```python
from build123d import *

# Parameters (mm, degrees)
SKETCH2_W     = 2.75
SKETCH2_H     = 10
CHAMFER1_SIZE = 3
CHAMFER2_SIZE = 1


with BuildPart() as part:
    # Sketch2 → Revolve1 (revolve)
    with BuildSketch(Plane(origin=(0, 0, 0), x_dir=(0, 0, -1), z_dir=(1, 0, 0))):
        Polygon((14.3, 12), (14.3, 0), (17.05, 0), (23.05, 0), (23.05, 12), align=None)
        with Locations((15.675, -5)):
            Rectangle(SKETCH2_W, SKETCH2_H)
    revolve(axis=Axis((0, -11.25, 0), (0, 1, 0)))

    # Chamfer1
    chamfer1_edges = [part.edges().sort_by_distance(p)[0] for p in [
        (0, 12, 23.05),
        (0, 0, 23.05),
    ]]
    chamfer(chamfer1_edges, length=CHAMFER1_SIZE)

    # Chamfer2
    chamfer2_edges = [part.edges().sort_by_distance(p)[0] for p in [
        (0, -10, 17.05),
    ]]
    chamfer(chamfer2_edges, length=CHAMFER2_SIZE)


solid = part.part
```
Build history of the part. All positions in model axes, mm. A direction names the side the tool comes from. Give positions to 0.01 mm unless a question says otherwise; leave off trailing zeros. Loops run counter-clockwise (first coordinate to the right, second up) from the corner with the lowest first, then second, coordinate; pieces in that order, holes last.
Item 1: Slice it at B-B, the plane x = 0. List the corners of the cut face in (y, z).
Answers follow:
outline: (-10, -16.05) - (-9, -17.05) - (0, -17.05) - (0, -20.05) - (3, -23.05) - (9, -23.05) - (12, -20.05) - (12, -14.3) - (-10, -14.3) - close; (-10, 14.3) - (12, 14.3) - (12, 20.05) - (9, 23.05) - (3, 23.05) - (0, 20.05) - (0, 17.05) - (-9, 17.05) - (-10, 16.05) - close
Item 2: Which spindle directions (+Z, -Z, +X, -X, +Y, -Y) get a long thin tool onto all of the face, cutting with end or side? Do faces 4 (the face through (-16.905, -4.437, 2.22)), 5 (the face through (11, -10, -10)). Say none if no direction does.
Answers follow:
face 4: -Y
face 5: +Z, -Z, +X, -X, -Y
Item 3: Slice it at C-C, the plane y = -2.25. List the corners of the cut face in (x, z), and give its area (3 significant figures).
Answers follow:
outline: circle Ø34.1 at (0, 0); hole circle Ø28.6 at (0, 0)
area: 271 mm2
Item 4: Flat gauge pins, fed straight in: pin 1 (12 mm diameter, centred on y = 1.5, z = 11.5, fed in from +X); pin 2 (1.5 mm diameter, centred on y = 2.5, z = 9.5, fed in from -X); pin 3 (4 mm diameter, centred on x = -3, z = 10.5, fed in from -Y); pin 4 (10 mm diameter, centred on x = 16, y = -3.5, fed in from -Z). Where does each tip first touch, or does it go through?
Answers follow:
pin 1: stops at x = 22.34
pin 2: stops at x = -21.25
pin 3: passes through
pin 4: stops at z = -15.94
Item 5: Pull direction X, two halves, no side cores. Call faces 1 (the face through (-16.4, 0, 5.8)), 2 (the face through (-14.18, 0.85, 1.86)), 3 (the face through (-15.578, 6.042, 16.989)): released by +X, released by -X, zero draft, split by the parting line, or undercut.
Answers follow:
face 1: zero draft
face 2: undercut
face 3: split by the parting line
Item 6: Slice it at A-A, the plane z = 0. List the corners of the cut face in (x, y).
Answers follow:
outline: (-23.05, 3) - (-20.05, 0) - (-17.05, 0) - (-17.05, -9) - (-16.05, -10) - (-14.3, -10) - (-14.3, 12) - (-20.05, 12) - (-23.05, 9) - close; (14.3, -10) - (16.05, -10) - (17.05, -9) - (17.05, 0) - (20.05, 0) - (23.05, 3) - (23.05, 9) - (20.05, 12) - (14.3, 12) - close
Item 7: Drill centre lines: line 1 (X direction, y = -4.25, z = 0); line 2 (Z direction, x = 0, y = 3). Where is each one in solid material? Low to high.
Answers follow:
line 1: x = -17.05 to -14.3, 14.3 to 17.05
line 2: z = -23.05 to -14.3, 14.3 to 23.05
